```python
from build123d import *

# Parameters (mm, degrees)
F0_W     = 165.1
F0_H     = 19.05
F1_DEPTH = 590.55
F2_W     = 165.1
F2_H     = 6.35
F3_DEPTH = 9.525
F4_W     = 165.1
F4_H     = 6.35
F5_DEPTH = 9.525


with BuildPart() as f1:
    # F0 (on Right) → F1 (new body)
    with BuildSketch(Plane.YZ):
        with Locations((82.55, 9.525)):
            Rectangle(F0_W, F0_H)
    extrude(amount=F1_DEPTH)

    # F2 (on face) → F3 (cut)
    with BuildSketch(Plane.YZ.offset(590.55)):
        with Locations((82.55, 3.175)):
            Rectangle(F2_W, F2_H)
    extrude(amount=-F3_DEPTH, mode=Mode.SUBTRACT)

    # F4 (on face) → F5 (cut)
    with BuildSketch(Plane(origin=(0, 0, 0), x_dir=(0, -1, 0), z_dir=(-1, 0, 0))):
        with Locations((-82.55, 3.175)):
            Rectangle(F4_W, F4_H)
    extrude(amount=-F5_DEPTH, mode=Mode.SUBTRACT)


solid = f1.part
```
Can you work these out from the model? Positions are in its coordinate system, mm. A direction names the side the tool comes from. Coordinates: 2 decimals unless noted, no trailing zeros. Answer as CSV lines item,"result".
Item 1: On a 3-axis mill with a long thin cutter (end or side, diameter ignored), from which of +Z, -Z, +X, -X, +Y, -Y can I reach the whole of each face in a straight line? I mean faces 1 (the flat face through (590.55, 81, 13)), 2 (the flat face through (5, 84, 6.35)), 3 (the flat face through (586, 81, 6.35)). Say none if no direction works.
Geometry results:
face 1,"+Z, -Z, +X, +Y, -Y"
face 2,"-Z, -X, +Y, -Y"
face 3,"-Z, +X, +Y, -Y"
Item 2: I'm going to push flat-ended pins straight in: P1, Ø3, axis at y = 72.5, z = 1.5, coming from the +X side (3 decimals); P2, Ø3, axis at y = 50.5, z = 1.5, coming from the -X side (3 decimals); P3, Ø3, axis at x = 587.5, y = 83.5, coming from the -Z side. Where does each tip first touch, or does it pass through?
Geometry results:
P1,"stops at x = 581.025"
P2,"stops at x = 9.525"
P3,"stops at z = 6.35"
Item 3: Please list where this line runs through material, in increasing order: line 1 along X through (y, z) = (108.5, 2.5) (3 decimals).
Geometry results:
line 1,"x = 9.525 to 581.025"
